```python
from build123d import *

# Parameters (mm, degrees)
BOSS_EXTRUDE1_DEPTH                          = 10
BOSS_EXTRUDE1_2_DEPTH                        = 10
CBORE_FOR_M5_HEX_SOCKET_HEAD_CAP_SCR_2_COUNT = 2
CBORE_FOR_M5_HEX_SOCKET_HEAD_CAP_SCR_2_PITCH = 30
BOSS_EXTRUDE2_DEPTH                          = 13
BOSS_EXTRUDE3_DEPTH                          = 23
BOSS_EXTRUDE4_DEPTH                          = 27
SKETCH8_R                                    = 2.1
CUT_EXTRUDE1_DEPTH                           = 52.298148115
CHAMFER1_SIZE                                = 16
CUT_EXTRUDE2_DEPTH                           = 6
SKETCH10_R                                   = 5
SKETCH10_R_2                                 = 2.1
BOSS_EXTRUDE5_DEPTH                          = 0.7
CHAMFER2_SIZE                                = 1


with BuildPart() as part:
    # Sketch1 → Boss-Extrude1 (new, symmetric)
    with BuildSketch(Plane.XY):
        with BuildLine():
            Line((-14, 32.5), (-1.5, 32.5))
            Line((-1.5, 32.5), (-1.5, 5.809475019))
            ThreePointArc((-1.5, 5.809475019), (-6, 0), (-1.5, -5.809475019))
            Line((-1.5, -5.809475019), (-1.5, -24.5))
            Line((-1.5, -24.5), (-14, -24.5))
            Line((-14, -24.5), (-14, 32.5))
        make_face()
    extrude(amount=BOSS_EXTRUDE1_DEPTH, both=True)


with BuildPart() as body_2:
    # Sketch1 → Boss-Extrude1 2 (new, symmetric)
    with BuildSketch(Plane.XY):
        with BuildLine():
            Line((15, 33.5), (15, 23))
            Line((15, 23), (15.6, 23))
            Line((15.6, 23), (15.6, 15))
            Line((15.6, 15), (15, 15))
            Line((15, 15), (15, -7))
            Line((15, -7), (15.6, -7))
            Line((15.6, -7), (15.6, -15))
            Line((15.6, -15), (15, -15))
            Line((15, -15), (15, -25.5))
            Line((15, -25.5), (1.5, -25.5))
            Line((1.5, -25.5), (1.5, -5.809475019))
            ThreePointArc((1.5, -5.809475019), (6, 0), (1.5, 5.809475019))
            Line((1.5, 5.809475019), (1.5, 33.5))
            Line((1.5, 33.5), (15, 33.5))
        make_face()
    extrude(amount=BOSS_EXTRUDE1_2_DEPTH, both=True)


with BuildPart() as cbore_for_m5_hex_socket_head_cap_screw1_tool:
    # Sketch2 → CBORE for M5 Hex Socket Head Cap Screw1 (revolve)
    with BuildSketch(Plane(origin=(-14, -11, 0), x_dir=(0, 0, 1), z_dir=(0, 1, 0))):
        Polygon((0, 0), (0, 29.6), (2.25, 29.6), (2.25, 5.9), (5, 5.9), (5, 0), align=None)
    cbore_for_m5_hex_socket_head_cap_screw1 = revolve(axis=Axis((-20.35, -11, 0), (1, 0, 0)))


with BuildPart() as part_1:
    add(part.part)

    # CBORE for M5 Hex Socket Head Cap Screw1: cut by cbore_for_m5_hex_socket_head_cap_screw1_tool
    add(cbore_for_m5_hex_socket_head_cap_screw1_tool.part, mode=Mode.SUBTRACT)


with BuildPart() as body_2_1:
    add(body_2.part)

    # CBORE for M5 Hex Socket Head Cap Screw1: cut by cbore_for_m5_hex_socket_head_cap_screw1_tool
    add(cbore_for_m5_hex_socket_head_cap_screw1_tool.part, mode=Mode.SUBTRACT)


with BuildPart() as cbore_for_m5_hex_socket_head_cap_scr_2_tool:
    # CBORE for M5 Hex Socket Head Cap Scr 2: CBORE for M5 Hex Socket Head Cap Screw1 ×2
    with Locations(*[(0, i * CBORE_FOR_M5_HEX_SOCKET_HEAD_CAP_SCR_2_PITCH, 0) for i in range(1, CBORE_FOR_M5_HEX_SOCKET_HEAD_CAP_SCR_2_COUNT)]):
        add(cbore_for_m5_hex_socket_head_cap_screw1)


with BuildPart() as part_2:
    add(part_1.part)

    # CBORE for M5 Hex Socket Head Cap Scr 2: cut by cbore_for_m5_hex_socket_head_cap_scr_2_tool
    add(cbore_for_m5_hex_socket_head_cap_scr_2_tool.part, mode=Mode.SUBTRACT)


with BuildPart() as body_2_2:
    add(body_2_1.part)

    # CBORE for M5 Hex Socket Head Cap Scr 2: cut by cbore_for_m5_hex_socket_head_cap_scr_2_tool
    add(cbore_for_m5_hex_socket_head_cap_scr_2_tool.part, mode=Mode.SUBTRACT)

    # Sketch4 → Boss-Extrude2 (add)
    with BuildSketch(Plane.XY.offset(10)):
        Polygon((1.5, 5.809475019), (1.5, -5.809475019), (1.5, -25.5), (15, -25.5), (15, -15), (15.6, -15), (15.6, -7), (15, -7), (15, 15), (15.6, 15), (15.6, 23), (15, 23), (15, 33.5), (1.5, 33.5), align=None)
    extrude(amount=BOSS_EXTRUDE2_DEPTH)

    # Sketch5 → Boss-Extrude3 (add)
    with BuildSketch(Plane(origin=(0, 0, -10), x_dir=(-1, 0, 0), z_dir=(0, 0, -1))):
        with BuildLine():
            Line((-15, -25.5), (-1.5, -25.5))
            Line((-1.5, -25.5), (-1.5, -5.809475019))
            ThreePointArc((-1.5, -5.809475019), (-6, 0), (-1.5, 5.809475019))
            Line((-1.5, 5.809475019), (-1.5, 33.5))
            Line((-1.5, 33.5), (-15, 33.5))
            Line((-15, 33.5), (-15, 23))
            Line((-15, 23), (-15.6, 23))
            Line((-15.6, 23), (-15.6, 15))
            Line((-15.6, 15), (-15, 15))
            Line((-15, 15), (-15, -7))
            Line((-15, -7), (-15.6, -7))
            Line((-15.6, -7), (-15.6, -15))
            Line((-15.6, -15), (-15, -15))
            Line((-15, -15), (-15, -25.5))
        make_face()
    extrude(amount=BOSS_EXTRUDE3_DEPTH)

    # Sketch7 → Boss-Extrude4 (add)
    with BuildSketch(Plane(origin=(0, 33.5, 0), x_dir=(1, 0, 0), z_dir=(0, 1, 0))):
        Polygon((1.5, 33), (-4.9, 33), (-4.9, 17.4), (1.5, 11), align=None)
    extrude(amount=-BOSS_EXTRUDE4_DEPTH)

    # Sketch8 → Cut-Extrude1 (cut, through all)
    with BuildSketch(Plane.ZY.offset(4.9)):
        with Locations((-25, 19)):
            Circle(SKETCH8_R)
    extrude(amount=-CUT_EXTRUDE1_DEPTH, mode=Mode.SUBTRACT)

    # Chamfer1
    chamfer1_edges = [body_2_2.edges().sort_by_distance(p)[0] for p in [
        (8.25, -25.5, -33),
    ]]
    chamfer(chamfer1_edges, length=CHAMFER1_SIZE)

    # Sketch9 → Cut-Extrude2 (cut)
    with BuildSketch(Plane(origin=(15.6, 0, 0), x_dir=(0, 0, -1), z_dir=(1, 0, 0))):
        Polygon((29.099186911, 19), (27.049593456, 22.55), (22.950406544, 22.55), (20.900813089, 19), (22.950406544, 15.45), (27.049593456, 15.45), align=None)
    extrude(amount=-CUT_EXTRUDE2_DEPTH, mode=Mode.SUBTRACT)

    # Sketch10 → Boss-Extrude5 (add)
    with BuildSketch(Plane.ZY.offset(4.9)):
        with Locations((-25, 19)):
            Circle(SKETCH10_R)
        with Locations((-25, 19)):
            Circle(SKETCH10_R_2, mode=Mode.SUBTRACT)
    extrude(amount=BOSS_EXTRUDE5_DEPTH)

    # Chamfer2
    # the kernel refuses this chamfer: 1 mm, written as the material it takes off along each edge
    with BuildSketch(Plane(origin=(-5.6, 19, -25), x_dir=(0, 0, 1), z_dir=(0, -1, 0))) as chamfer2_piece_1_section:
        Polygon((5, -CHAMFER2_SIZE), (5 - CHAMFER2_SIZE, 0), (5, 0), align=None)
    chamfer2_piece_1 = revolve(axis=Axis((-5.6, 19, -25), (-1, 0, 0)), mode=Mode.PRIVATE)
    chamfer2_piece_1 = split(chamfer2_piece_1, bisect_by=Plane(origin=(-4.9, 19, -29.353058273), z_dir=(-1, 0, 0)), keep=Keep.TOP, mode=Mode.PRIVATE)
    add(chamfer2_piece_1, mode=Mode.SUBTRACT)


solid = part_2.part
```
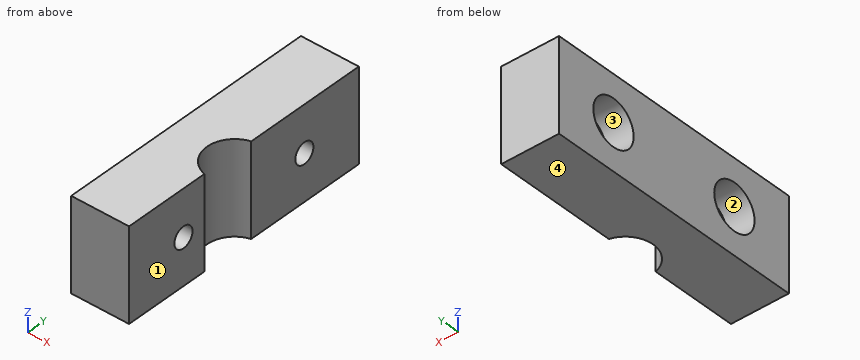
The listing builds one solid part. Answer for the finished solid, in the listing's coordinates (mm). Face numbers are marked on the shaded views. Round coordinates to 2 decimals unless told otherwise and drop trailing zeros. Write each loop counter-clockwise with the first axis right and the second up, starting at its lowest first coordinate (ties: lowest second). Pieces come first, ordered by that corner, then holes. Notation, with made-up numbers: (-23, -31.5) -> (21, -31.5) arc R21 cw to (21, -18.5) -> close; hole circle Ø10 at (-5.5, 15.5). An arc over 180 degrees is marked (long way). Use CSV: the item, a comma, the result in double quotes. Start each with the question number.
(1) The mould has two halves that part along Z. Classify the marked faces 1, 2, 3 and 4: released by +Z, released by -Z, zero draft, split by the parting line, or undercut.
(2) Section A-A on z = 0 is taken. Give the vertices of the cut face in (x, y).
(3) Section D-D on z = 4 is taken. Give the vertices of the cut face in (x, y), then the cut area to 3 significant figures.
(4) Consider L1, parallel to Z at x = -10.25, y = 19; L2, parallel to Z at x = -2.25, y = 19; L3, parallel to Y at x = -8.25, z = -3. Determine where each line is inside the solid, lowest interval first. Write a range as from..to.
(5) Each of these flat-tipped pins is pushed along its axis until it touches: pin 1 (3 mm diameter, centred on y = -9, z = 0, fed in from -X); pin 2 (4 mm diameter, centred on y = -11, z = 0, fed in from +X). Where does it stop, or does it pass through?
(6) Section B-B on y = 19 is taken. Give the vertices of the cut face in (x, z), then the cut area to 3 significant figures.
(7) Section C-C on x = -6.5 is taken. Give the vertices of the cut face in (y, z).
A:
1,face 1,"zero draft"
1,face 2,"undercut"
1,face 3,"undercut"
1,face 4,"released by -Z"
2,outline,"(-14, -24.5) -> (-1.5, -24.5) -> (-1.5, -13.25) -> (-8.1, -13.25) -> (-8.1, -16) -> (-14, -16) -> close; (-14, -6) -> (-8.1, -6) -> (-8.1, -8.75) -> (-1.5, -8.75) -> (-1.5, -5.81) arc R6 cw to (-1.5, 5.81) -> (-1.5, 16.75) -> (-8.1, 16.75) -> (-8.1, 14) -> (-14, 14) -> close; (-14, 24) -> (-8.1, 24) -> (-8.1, 21.25) -> (-1.5, 21.25) -> (-1.5, 32.5) -> (-14, 32.5) -> close"
3,outline,"(-14, -24.5) -> (-1.5, -24.5) -> (-1.5, -5.81) arc R6 cw to (-1.5, 5.81) -> (-1.5, 32.5) -> (-14, 32.5) -> (-14, 22) -> (-8.1, 22) -> (-8.1, 16) -> (-14, 16) -> (-14, -8) -> (-8.1, -8) -> (-8.1, -14) -> (-14, -14) -> close"
3,area,"603 mm²"
4,L1,"z = -10..-5, 5..10"
4,L2,"z = -10..-2.25, 2.25..10"
4,L3,"y = -24.5..-15, -7..15, 23..32.5"
5,pin 1,"stops at x = -8.1"
5,pin 2,"passes through"
6,outline,"(-14, -10) -> (-1.5, -10) -> (-1.5, -2.25) -> (-8.1, -2.25) -> (-8.1, -5) -> (-14, -5) -> close; (-14, 5) -> (-8.1, 5) -> (-8.1, 2.25) -> (-1.5, 2.25) -> (-1.5, 10) -> (-14, 10) -> close"
6,area,"161 mm²"
7,outline,"(-24.5, -10) -> (32.5, -10) -> (32.5, 10) -> (-24.5, 10) -> close; hole circle Ø4.5 at (-11, 0); hole circle Ø4.5 at (19, 0)"
